Autodesk Inventor part; units mm, degrees
ref_plane "YZ Plane" through (0, 0, 0) normal (1, 0, 0) x (0, 1, 0)
ref_plane "XZ Plane" through (0, 0, 0) normal (0, 1, 0) x (-1, 0, 0)
ref_plane "XY Plane" through (0, 0, 0) normal (0, 0, 1) x (1, 0, 0)
sketch "main" plane through (0, 0, 0) normal (0, 0, 1) x (1, 0, 0)
  line L0 (12.0188, -14.2552) -> (37.3756, 32.0398)
  circle A0 centre (21.7688, 21.6141) radius 2.1844
  line L1 (40.1954, 36.1649) -> (45.6883, 42.7111)
  circle A1 centre (31.8098, 33.5805) radius 2.1844
  circle A2 centre (36.488, 51.5844) radius 2.1844
  arc A3 (42.4433, 53.7882) -> (36.4888, 57.9344) centre (36.488, 51.5844) ccw
  line L2 (45.961, 44.2825) -> (42.4433, 53.7882)
  arc A4 (45.6883, 42.7111) -> (45.961, 44.2825) centre (44.4722, 43.7316) ccw
  line L3 (36.4888, 57.9344) -> (-17.6519, 57.9412)
  circle A5 centre (7.7473, 51.5844) radius 2.1844
  line L4 (7.7515, 35.7094) -> (7.7532, 29.3619)
  arc A6 (7.7515, 35.7094) -> (-1.776, 45.2318) centre (-1.7735, 35.7068) ccw
  arc A7 (-1.7718, 19.8344) -> (7.7532, 29.3619) centre (-1.7718, 29.3594) ccw
  line L5 (-17.651, 45.2276) -> (-1.776, 45.2318)
  arc A8 (-17.6519, 57.9412) -> (-17.651, 45.2276) centre (-17.6527, 51.5844) ccw
  arc A9 (-17.6527, 19.8344) -> (-21.9541, 8.8131) centre (-17.6527, 13.4844) ccw
  circle A10 centre (7.7473, 13.4844) radius 2.1844
  line L6 (-1.7718, 19.8344) -> (-17.6527, 19.8344)
  arc A11 (4.4483, -15.4983) -> (12.0188, -14.2552) centre (7.7473, -11.9156) ccw
  line L7 (4.4483, -15.4983) -> (-21.9541, 8.8131)
  circle A12 centre (7.7473, -11.9156) radius 2.1844
  circle A13 centre (-17.6527, 51.5844) radius 2.1844
  circle A14 centre (-17.6527, 13.4844) radius 2.1844
  arc A15 (40.1954, 36.1649) -> (37.3756, 32.0398) centre (59.6529, 19.8381) ccw
  point P0 (10.5119, 26.5593)
  dimension "d1" = 9.7405
  dimension "d2" = 4.3688
  dimension "d3" = 4.3688
  dimension "d4" = 4.3688
  dimension "d5" = 4.3688
  dimension "d6" = 4.3688
  dimension "d7" = 25.4
sketch "Sketch1" plane through (0, 0, 0) normal (0, 1, 0) x (-1, 0, 0)
  line L0 (29.6715, -65.8396) -> (55.0283, -19.5445)
  circle A0 centre (39.4215, -29.9702) radius 2.1844
  line L1 (57.8481, -15.4195) -> (63.341, -8.8732)
  circle A1 centre (49.4625, -18.0039) radius 2.1844
  circle A2 centre (54.1407, 0) radius 2.1844
  arc A3 (60.096, 2.2039) -> (54.1415, 6.35) centre (54.1407, 0) ccw
  line L2 (63.6138, -7.3019) -> (60.096, 2.2039)
  arc A4 (63.341, -8.8732) -> (63.6138, -7.3019) centre (62.1249, -7.8528) ccw
  line L3 (54.1415, 6.35) -> (0.0008, 6.3568)
  circle A5 centre (25.4, 0) radius 2.1844
  line L4 (25.4043, -15.875) -> (25.406, -22.2224)
  arc A6 (25.4043, -15.875) -> (15.8767, -6.3526) centre (15.8793, -15.8776) ccw
  arc A7 (15.881, -31.75) -> (25.406, -22.2224) centre (15.881, -22.225) ccw
  line L5 (0.0017, -6.3568) -> (15.8767, -6.3526)
  arc A8 (0.0008, 6.3568) -> (0.0017, -6.3568) centre (0, 0) ccw
  arc A9 (0, -31.75) -> (-4.3013, -42.7713) centre (0, -38.1) ccw
  circle A10 centre (25.4, -38.1) radius 2.1844
  line L6 (15.881, -31.75) -> (0, -31.75)
  arc A11 (22.101, -67.0827) -> (29.6715, -65.8396) centre (25.4, -63.5) ccw
  line L7 (22.101, -67.0827) -> (-4.3013, -42.7713)
  circle A12 centre (25.4, -63.5) radius 2.1844
  circle A13 centre (0, 0) radius 2.1844
  circle A14 centre (0, -38.1) radius 2.1844
  arc A15 (57.8481, -15.4195) -> (55.0283, -19.5445) centre (77.3056, -31.7463) ccw
extrude "Extrusion1" add sketch "Sketch1" along normal blind 1.5875
properties part number "Funnel Gusset Back Improved" material "Acetal Resin, White"
Source: CAD feature listing. Evaluate the final solid. Frame: model axes, mm. A direction names the side the tool comes from. Give positions to 0.01 mm unless a question says otherwise; leave off trailing zeros. Order: outer loops, then holes, each group sorted by start corner. A loop starts at its lowest first (then second) coordinate and runs counter-clockwise, first axis right, second up. Notation, with made-up numbers: (4, 58.5) -> (22, 58.5) arc R9 cw to (22, 62.5) -> close; hole circle Ø11 at (78.25, -2). An arc over 180 degrees is marked (long way). Write item = value, one per line.
Q1. Pull-direction query (X, two-part tool) for faces 1 (the face through (-56.159, 0.783, 0.837)), 2 (the face through (-9.085, 0.783, -55.097)), 3 (the face through (-26.25, 0.783, -68.295)), 4 (the face through (-42.17, 0.78, -43.02)); classes: released by +X, released by -X, zero draft, split by the parting line, or undercut.
Data:
face_1 = undercut
face_2 = released by +X
face_3 = split by the parting line
face_4 = released by -X
Q2. Cut plane A-A, the plane z = 0. Output: boundary loops of the cut face in (x, y).
Data:
outline = (-60.91, 0) -> (-56.33, 0) -> (-56.33, 1.59) -> (-60.91, 1.59) -> close; (-51.96, 0) -> (-27.58, 0) -> (-27.58, 1.59) -> (-51.96, 1.59) -> close; (-23.22, 0) -> (-2.18, 0) -> (-2.18, 1.59) -> (-23.22, 1.59) -> close; (2.18, 0) -> (6.36, 0) -> (6.36, 1.59) -> (2.18, 1.59) -> close
Q3. Cut plane B-B, the plane y = 0.5. State how many separate pieces and enclosed holes the cut face has, and give its area (3 significant figures).
Data:
separate_pieces = 1
enclosed_holes = 8
area = 2,740 mm^2
Q4. Pin query (flat end, axial travel): pin 1 (0.5 mm diameter, centred on y = 0.5, z = -19, fed in from +X). Return the tip coordinate at first contact, or that it passes through.
Data:
pin_1 = -25.41
Q5. Cut plane D-D, the plane x = -10. Output: boundary loops of the cut face in (y, z).
Data:
outline = (0, -55.94) -> (1.59, -55.94) -> (1.59, -31.75) -> (0, -31.75) -> close; (0, -6.35) -> (1.59, -6.35) -> (1.59, 6.36) -> (0, 6.36) -> close
Q6. Material intervals for line 1 (Z direction, x = 0, y = 0.85); line 2 (X direction, y = 1.3, z = -2); line 3 (Z direction, x = 1.5, y = 0.85), sorted ascending. Write a range as from..to.
Data:
line_1 = -46.73..-40.28, -35.92..-31.75, -6.36..-2.18, 2.18..6.36
line_2 = -61.65..-55.02, -53.26..-26.28, -24.52..-0.88, 0.88..6.03
line_3 = -45.35..-39.69, -36.51..-31.93, -6.18..-1.59, 1.59..6.18
Q7. Cut plane C-C, the plane x = -38.5. Output: boundary loops of the cut face in (y, z).
Data:
outline = (0, -49.72) -> (1.59, -49.72) -> (1.59, -31.95) -> (0, -31.95) -> close; (0, -27.99) -> (1.59, -27.99) -> (1.59, 6.35) -> (0, 6.35) -> close
Q8. Set-up query: faces 5 (the face through (-22.691, 0.783, -28.885)), 6 (the face through (-57.725, 0.783, 5.242)). Return all of +Z, -Z, +X, -X, +Y, -Y with unobstructed straight access to the full face (end or side cutting, diameter ignored); none if empty.
Data:
face_5 = +X, +Y, -Y
face_6 = +Z, -X, +Y, -Y
